```python
from build123d import *

# Parameters (mm, degrees)
SKETCH_1_W          = 60
SKETCH_1_H          = 42
EXTRUDE_1_DEPTH     = 3
CUT_EXTRUDE_1_DEPTH = 3
FILLET_1_R          = 3


with BuildPart() as part:
    # 草图1 → 凸台-拉伸1 (new body)
    with BuildSketch(Plane.XY):
        Rectangle(SKETCH_1_W, SKETCH_1_H)
    extrude(amount=EXTRUDE_1_DEPTH)

    # 草图2 → 切除-拉伸1 (cut)
    with BuildSketch(Plane.XY.offset(3)):
        with BuildLine():
            Line((-23.5, 18.25), (-20.5, 18.25))
            ThreePointArc((-20.5, 18.25), (-17.25, 15), (-20.5, 11.75))
            Line((-20.5, 11.75), (-23.5, 11.75))
            ThreePointArc((-23.5, 11.75), (-26.75, 15), (-23.5, 18.25))
        make_face()
        with BuildLine():
            Line((20.5, 18.25), (23.5, 18.25))
            ThreePointArc((23.5, 18.25), (26.75, 15), (23.5, 11.75))
            Line((23.5, 11.75), (20.5, 11.75))
            ThreePointArc((20.5, 11.75), (17.25, 15), (20.5, 18.25))
        make_face()
        with BuildLine():
            Line((20.5, -18.25), (23.5, -18.25))
            ThreePointArc((23.5, -18.25), (26.75, -15), (23.5, -11.75))
            Line((23.5, -11.75), (20.5, -11.75))
            ThreePointArc((20.5, -11.75), (17.25, -15), (20.5, -18.25))
        make_face()
        with BuildLine():
            Line((-23.5, -18.25), (-20.5, -18.25))
            ThreePointArc((-20.5, -18.25), (-17.25, -15), (-20.5, -11.75))
            Line((-20.5, -11.75), (-23.5, -11.75))
            ThreePointArc((-23.5, -11.75), (-26.75, -15), (-23.5, -18.25))
        make_face()
    extrude(amount=-CUT_EXTRUDE_1_DEPTH, mode=Mode.SUBTRACT)

    # 圆角1
    fillet_1_edges = [part.edges().sort_by_distance(p)[0] for p in [
        (-30, 21, 1.5),
        (30, 21, 1.5),
        (30, -21, 1.5),
        (-30, -21, 1.5),
    ]]
    fillet(fillet_1_edges, radius=FILLET_1_R)


solid = part.part
```
Input: part model. Units: mm. Frame: model coordinates. A direction names the side the tool comes from. Give positions to 0.01 mm unless a question says otherwise; leave off trailing zeros. Order: outer loops, then holes, each group sorted by start corner. A loop starts at its lowest first (then second) coordinate and runs counter-clockwise, first axis right, second up. Notation, with made-up numbers: M -13,82.5 L 35,82.5 A4 cw 35,89.5 Z; hole C 14.5,44.25 d9. An arc over 180 degrees is marked long. Return JSON: item names as keys, results as strings.
Item 1: Ray query, probe 1 along Y at (x, z) = (-23.5, 2.25); probe 2 along X at (y, z) = (-16, 1); probe 3 along X at (y, z) = (15.5, 0.25). Return the intervals inside material, ascending.
Solutions:
{"probe 1": "-21 to -18.25, -11.75 to 11.75, 18.25 to 21", "probe 2": "-30 to -26.59, -17.41 to 17.41, 26.59 to 30", "probe 3": "-30 to -26.71, -17.29 to 17.29, 26.71 to 30"}
Item 2: Cut plane A-A (z = 0.75). Return loops of the section in (x, y), then the cut area to 3 significant figures.
Solutions:
{"outline": "M -30,-18 A3 ccw -27,-21 L 27,-21 A3 ccw 30,-18 L 30,18 A3 ccw 27,21 L -27,21 A3 ccw -30,18 Z; hole M -23.5,-18.25 L -20.5,-18.25 A3.25 ccw -20.5,-11.75 L -23.5,-11.75 A3.25 ccw Z; hole M -23.5,11.75 L -20.5,11.75 A3.25 ccw -20.5,18.25 L -23.5,18.25 A3.25 ccw Z; hole M 20.5,-18.25 L 23.5,-18.25 A3.25 ccw 23.5,-11.75 L 20.5,-11.75 A3.25 ccw Z; hole M 20.5,11.75 L 23.5,11.75 A3.25 ccw 23.5,18.25 L 20.5,18.25 A3.25 ccw Z", "area": "2,300 mm^2"}
Item 3: Cut plane B-B (y = 15). Return loops of the section in (x, z), then the cut area to 3 significant figures.
Solutions:
{"outline": "M -30,0 L -26.75,0 L -26.75,3 L -30,3 Z; M -17.25,0 L 17.25,0 L 17.25,3 L -17.25,3 Z; M 26.75,0 L 30,0 L 30,3 L 26.75,3 Z", "area": "123 mm^2"}
Item 4: Pull-direction query (X, two-part tool) for faces 1 (the cylindrical face through (-29.14, -20.1, 1.52)), 2 (the flat face through (0, -21, 1)), 3 (the flat face through (-22, -11.75, 2)); classes: +X half, -X half, draft (parallel to the pull), parting line (faces both ways), or undercut.
Solutions:
{"face 1": "-X half", "face 2": "draft", "face 3": "undercut"}
Item 5: Access query for faces 4 (the cylindrical face through (-29.14, 20.1, 1.52)), 5 (the cylindrical face through (17.25, -14.93, 1.52)). Directions: +Z, -Z, +X, -X, +Y, -Y. A direction counts if a zero-diameter tool reaches every point of the face in a straight line with its end or side. Return the directions, or none.
Solutions:
{"face 4": "+Z, -Z, -X, +Y", "face 5": "+Z, -Z"}
